Design review of the part shown in the three views and the two pictorial views. Dimensions are in mm from the part's minimum x, y and z. A direction names the side the tool comes from. Round coordinates to 2 decimals unless told otherwise and drop trailing zeros. Order: outer loops, then holes, each group sorted by start corner. A loop starts at its lowest first (then second) coordinate and runs counter-clockwise, first axis right, second up. Notation, with made-up numbers: (50, -36) - (102, -36) arc R6 ccw to (102, -26) - close; hole circle Ø7 at (74, 22). An arc over 180 degrees is marked (long way). One line per item, written item: value.
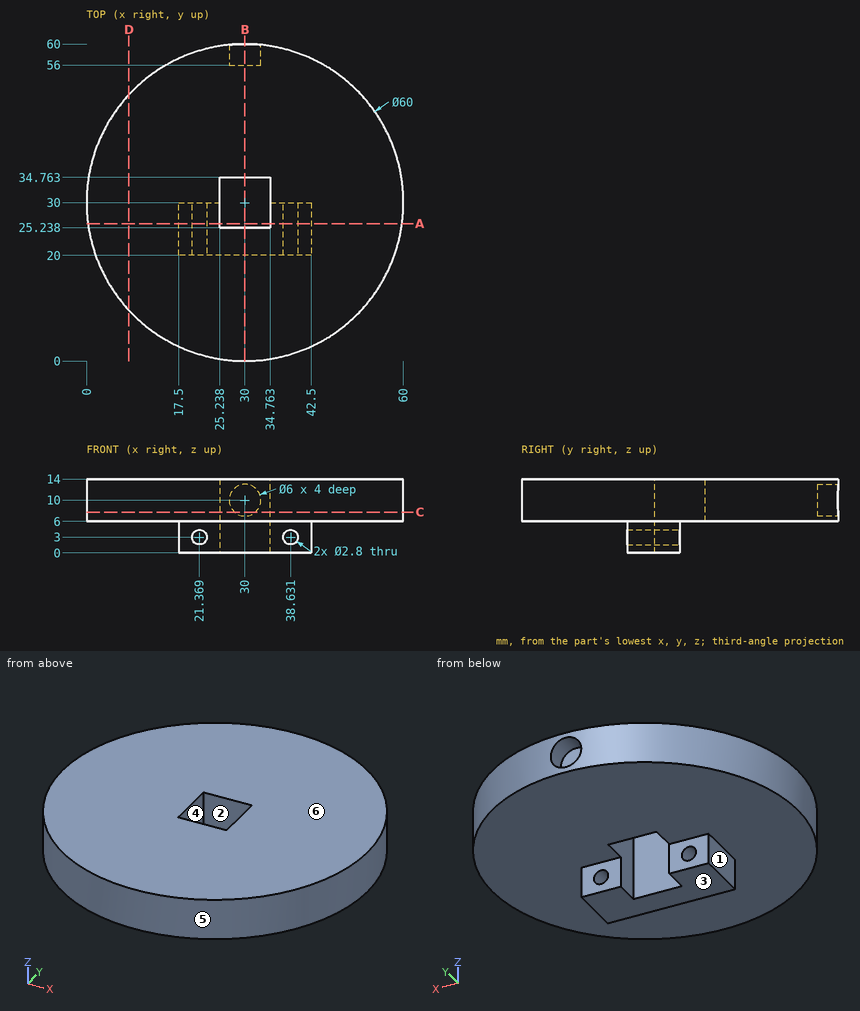
Item 1: The part is to be moulded in two halves that separate along Y. For the marked faces 4, 5 and 6, say which applies: +Y half, -Y half, draft (parallel to the pull), parting line (faces both ways), or undercut.
Returned:
face 4: undercut
face 5: parting line
face 6: draft
Item 2: Wall thickness on line 1 (X direction, y = 24.5, z = 3); line 2 (X direction, y = 26.25, z = 3); line 3 (Y direction, x = 30, z = 9): over which ranges is each line inside the solid? List them lowest first.
Returned:
line 1: 17.5 to 19.97, 22.77 to 37.23, 40.03 to 42.5
line 2: 17.5 to 19.97, 22.77 to 25.24, 34.76 to 37.23, 40.03 to 42.5
line 3: 0 to 25.24, 34.76 to 56
Item 3: For P1, Ø3, axis at y = 27, z = 3, coming from the -X side; P2, Ø1.5, axis at y = 25.5, z = 2, coming from the +X side; P3, Ø3, axis at x = 31, z = 10.5, coming from the +Y side, all flat-tipped, find the tip position at first contact; note any pin that passes through.
Returned:
P1: x = 17.5
P2: x = 42.5
P3: y = 56
Item 4: Take a section at C-C (z = 7.75). Write out the cut boundary in (x, y) (1 decimal).
Returned:
outline: (28, 56) - (28, 59.9) arc R30 ccw (long way) to (32, 59.9) - (32, 56) - close; hole (25.2, 25.2) - (34.8, 25.2) - (34.8, 34.8) - (25.2, 34.8) - close
Item 5: Machinability: for the marked faces 1, 2 and 3, which of the approach directions +Z, -Z, +X, -X, +Y, -Y give a long, thin tool a straight path to every point of the face, cutting with its end or side? Answer none if there is none.
Returned:
face 1: -Z, -X, +Y, -Y
face 2: +Z, -Z
face 3: -Z, +X, -X, +Y, -Y
Item 6: Take a section at A-A (y = 26). Write out the cut boundary in (x, z), plus the area to 3 significant figures.
Returned:
outline: (0.27, 6) - (17.5, 6) - (17.5, 0) - (25.24, 0) - (25.24, 14) - (0.27, 14) - close; (34.76, 0) - (42.5, 0) - (42.5, 6) - (59.73, 6) - (59.73, 14) - (34.76, 14) - close; hole circle Ø2.8 at (21.37, 3); hole circle Ø2.8 at (38.63, 3)
area: 480 mm^2
Item 7: Take a section at B-B (x = 30). Write out the cut boundary in (y, z), plus the area to 3 significant figures.
Returned:
outline: (0, 6) - (20, 6) - (20, 0) - (25.24, 0) - (25.24, 14) - (0, 14) - close; (34.76, 6) - (60, 6) - (60, 7) - (56, 7) - (56, 13) - (60, 13) - (60, 14) - (34.76, 14) - close
area: 411 mm^2
Item 8: Take a section at D-D (x = 8). Write out the cut boundary in (y, z).
Returned:
outline: (9.6, 6) - (50.4, 6) - (50.4, 14) - (9.6, 14) - close
